Part model, mm, in its own coordinate system. A direction names the side the tool comes from. Round coordinates to 2 decimals unless told otherwise and drop trailing zeros. Loops run counter-clockwise (first coordinate to the right, second up) from the corner with the lowest first, then second, coordinate; pieces in that order, holes last. Notation, with made-up numbers: M -11.75,46.25 L 2.25,46.25 A20 ccw 2.25,68.25 Z; hole C 50.5,58.5 d8. An arc over 180 degrees is marked long. Put each result on its own line as item: value. Start each with the question number.
1) Slice it at B-B on x = 11.5. Give the cut face in (y, z).
2) Drop flat-ended pins along their axis: pin 1 Ø1.5 at (y, z) = (2.5, -51.5) entering from +X; pin 2 Ø1 at (y, z) = (1, -49) entering from +X; pin 3 Ø0.9 at (x, y) = (8.5, 2) entering from -Z. Give the stop position or say it passes through.
3) Slice it at C-C on z = -62.5. Give the cut face in (x, y), then the cut area to 3 significant figures.
4) Probe line 1 along Z through (x, y) = (9, 1.15); line 2 along Z through (x, y) = (5.5, 1.85); line 3 along X through (y, z) = (0.95, -78.5). List the from-to ranges inside material, lowest first.
5) Pull direction Z, two halves, no side cores. Call faces 1 (the flat face through (61.04, 1.48, -41.31)), 2 (the flat face through (9, 1, -3.4)), 3 (the cylindrical face through (19.735, 1.479, -13.782)): +Z half, -Z half, draft (parallel to the pull), parting line (faces both ways), or undercut.
6) Which spindle directions (+Z, -Z, +X, -X, +Y, -Y) get a long thin tool onto all of the face, cutting with end or side? Do faces 4 (the flat face through (2, 1, -3.4)), 5 (the flat face through (98.674, 1, -88)), 6 (the flat face through (7, 1, -13)), 7 (the flat face through (-2, 1, -10)). Say none if no direction does.
```python
from build123d import *

# Parameters (mm, degrees)
SALIENTE_EXTRUIR1_DEPTH = 3
REDONDEO1_R             = 1


with BuildPart() as part:
    # Croquis1 → Saliente-Extruir1 (new body)
    with BuildSketch(Plane(origin=(0, 0, 0), x_dir=(1, 0, 0), z_dir=(0, 1, 0))):
        with BuildLine():
            Line((10, 3.4), (7, 3.4))
            Line((7, 3.4), (7, 2))
            Line((7, 2), (3, 2))
            Line((3, 2), (3, 3.4))
            Line((3, 3.4), (0, 3.4))
            Line((0, 3.4), (0, 0))
            Line((0, 0), (15.585786438, 0))
            ThreePointArc((15.585786438, 0), (19.412620761, 0.761204675), (22.656854249, 2.928932188))
            Line((22.656854249, 2.928932188), (100.509667992, 80.781745931))
            ThreePointArc((100.509667992, 80.781745931), (102.677395505, 84.025979419), (103.43860018, 87.852813742))
            Line((103.43860018, 87.852813742), (103.43860018, 90.210678119))
            Line((103.43860018, 90.210678119), (98.67360018, 90.210678119))
            Line((98.67360018, 90.210678119), (98.67360018, 87.010678119))
            Line((98.67360018, 87.010678119), (95.47360018, 87.010678119))
            Line((95.47360018, 87.010678119), (95.47360018, 90.210678119))
            Line((95.47360018, 90.210678119), (90.710678119, 90.210678119))
            Line((90.710678119, 90.210678119), (90.710678119, 87.852813742))
            ThreePointArc((90.710678119, 87.852813742), (89.949473444, 84.025979419), (87.781745931, 80.781745931))
            Line((87.781745931, 80.781745931), (22.928932188, 15.928932188))
            ThreePointArc((22.928932188, 15.928932188), (19.6846987, 13.761204675), (15.857864376, 13))
            Line((15.857864376, 13), (-3, 13))
            Line((-3, 13), (-3, 10))
            Line((-3, 10), (0, 10))
            Line((0, 10), (0, 6.6))
            Line((0, 6.6), (3, 6.6))
            Line((3, 6.6), (3, 8))
            Line((3, 8), (7, 8))
            Line((7, 8), (7, 6.6))
            Line((7, 6.6), (10, 6.6))
            Line((10, 6.6), (10, 3.4))
        make_face()
    extrude(amount=SALIENTE_EXTRUIR1_DEPTH)

    # Redondeo1
    redondeo1_edges = [part.edges().sort_by_distance(p)[0] for p in [
        (90.710678119, 1.5, -90.210678119),
        (95.47360018, 1.5, -90.210678119),
        (98.67360018, 1.5, -90.210678119),
        (103.43860018, 1.5, -90.210678119),
    ]]
    fillet(redondeo1_edges, radius=REDONDEO1_R)


solid = part.part
```
Recorded:
1. outline: M 0,-13 L 3,-13 L 3,0 L 0,0 Z
2. pin 1: stops at x = 71.98
2. pin 2: stops at x = 69.23
2. pin 3: stops at z = -13
3. outline: M 69.5,0 L 82.23,0 L 82.23,3 L 69.5,3 Z
3. area: 38.2 mm2
4. line 1: z = -13 to -6.6, -3.4 to 0
4. line 2: z = -13 to -8, -2 to 0
4. line 3: x = 85.5 to 98.23
5. face 1: +Z half
5. face 2: undercut
5. face 3: -Z half
6. face 4: -X, +Y, -Y
6. face 5: -Z, +Y, -Y
6. face 6: -Z, -X, +Y, -Y
6. face 7: +Z, -X, +Y, -Y
